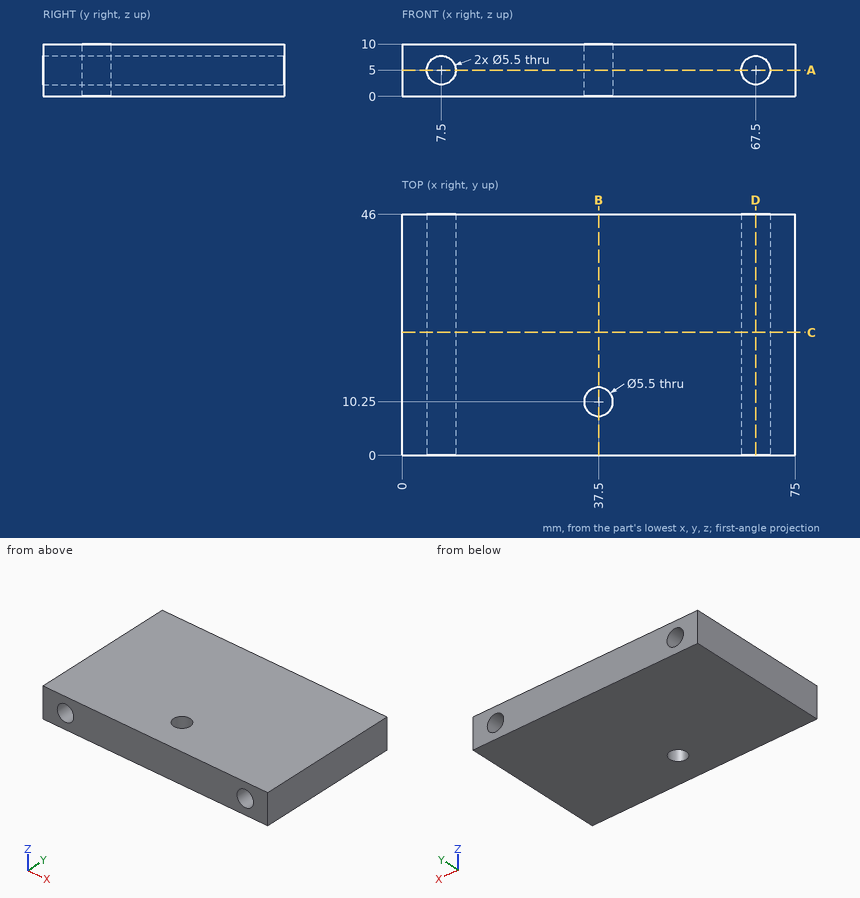
Source: three-view drawing plus pictorial views. Frame: mm from the lowest corner of the part. Give positions to 0.01 mm unless a question says otherwise; leave off trailing zeros. Write each loop counter-clockwise with the first axis right and the second up, starting at its lowest first coordinate (ties: lowest second). Pieces come first, ordered by that corner, then holes. Notation, with made-up numbers: (86, 84) - (143, 84) arc R30 cw to (143, 111) - close; hole circle Ø5 at (42, 69.25). An arc over 180 degrees is marked (long way). Write item = value, one per line. Start each with the question number.
Q1. Cut plane D-D, the plane x = 67.5. Return loops of the section in (y, z), then the cut area to 3 significant figures.
Q2. Material intervals for probe 1 along X at (y, z) = (31.5, 5); probe 2 along Y at (x, z) = (37.5, 7.5); probe 3 along X at (y, z) = (21, 3), sorted ascending.
Q3. Cut plane A-A, the plane z = 5. Return loops of the section in (x, y).
Q4. Cut plane B-B, the plane x = 37.5. Return loops of the section in (y, z).
Q5. Pin query (flat end, axial travel): pin 1 Ø3.5 at (x, y) = (37.5, 10.25) entering from +Z. Return the tip coordinate at first contact, or that it passes through.
Q6. Cut plane C-C, the plane y = 23.5. Return loops of the section in (x, z).
Computed values:
q1.outline = (0, 0) - (46, 0) - (46, 2.25) - (0, 2.25) - close; (0, 7.75) - (46, 7.75) - (46, 10) - (0, 10) - close
q1.area = 207 mm²
q2.probe_1 = 0 to 4.75, 10.25 to 64.75, 70.25 to 75
q2.probe_2 = 0 to 7.5, 13 to 46
q2.probe_3 = 0 to 5.61, 9.39 to 65.61, 69.39 to 75
q3.outline = (0, 0) - (4.75, 0) - (4.75, 46) - (0, 46) - close; (10.25, 0) - (64.75, 0) - (64.75, 46) - (10.25, 46) - close; (70.25, 0) - (75, 0) - (75, 46) - (70.25, 46) - close; hole circle Ø5.5 at (37.5, 10.25)
q4.outline = (0, 0) - (7.5, 0) - (7.5, 10) - (0, 10) - close; (13, 0) - (46, 0) - (46, 10) - (13, 10) - close
q5.pin_1 = through
q6.outline = (0, 0) - (75, 0) - (75, 10) - (0, 10) - close; hole circle Ø5.5 at (7.5, 5); hole circle Ø5.5 at (67.5, 5)
